from build123d import *

# Parameters (mm, degrees)
SKETCH_W        = 190
SKETCH_H        = 300
PAD_DEPTH       = 6.35
SKETCH001_R     = 2.75
POCKET_DEPTH    = 6.351
SKETCH002_R     = 4
SKETCH002_W     = 10
SKETCH002_H     = 4.75
SKETCH002_W_2   = 4.75
SKETCH002_H_2   = 10
POCKET001_DEPTH = 6.351
SKETCH003_R     = 4
POCKET002_DEPTH = 6.351
SKETCH004_R     = 2.5781
POCKET003_DEPTH = 6.351


with BuildPart() as part:
    # Sketch → Pad (new body)
    with BuildSketch(Plane.XY):
        with Locations((95, 150)):
            Rectangle(SKETCH_W, SKETCH_H)
    extrude(amount=PAD_DEPTH)

    # Sketch001 → Pocket (cut, through all)
    with BuildSketch(Plane.XY.offset(6.35)):
        with Locations((20, 280)):
            Circle(SKETCH001_R)
        with Locations((20, 240)):
            Circle(SKETCH001_R)
        with Locations((60, 240)):
            Circle(SKETCH001_R)
        with Locations((60, 280)):
            Circle(SKETCH001_R)
        with Locations((128, 280)):
            Circle(SKETCH001_R)
        with Locations((168, 280)):
            Circle(SKETCH001_R)
        with Locations((128, 240)):
            Circle(SKETCH001_R)
        with Locations((168, 240)):
            Circle(SKETCH001_R)
        with Locations((20, 55)):
            Circle(SKETCH001_R)
        with Locations((60, 55)):
            Circle(SKETCH001_R)
        with Locations((20, 15)):
            Circle(SKETCH001_R)
        with Locations((60, 15)):
            Circle(SKETCH001_R)
        with Locations((128, 15)):
            Circle(SKETCH001_R)
        with Locations((168, 55)):
            Circle(SKETCH001_R)
        with Locations((128, 55)):
            Circle(SKETCH001_R)
        with Locations((168, 15)):
            Circle(SKETCH001_R)
    extrude(amount=-POCKET_DEPTH, mode=Mode.SUBTRACT)

    # Sketch002 → Pocket001 (cut, through all)
    with BuildSketch(Plane(origin=(0, 0, 0), x_dir=(1, 0, 0), z_dir=(0, 0, -1))):
        with Locations((49.875, -148)):
            Circle(SKETCH002_R)
        with Locations((49.875, -192)):
            Circle(SKETCH002_R)
        with Locations((140.125, -148)):
            Circle(SKETCH002_R)
        with Locations((140.125, -192)):
            Circle(SKETCH002_R)
        with Locations((95, -122.375)):
            Rectangle(SKETCH002_W, SKETCH002_H)
        with Locations((95, -217.375)):
            Rectangle(SKETCH002_W, SKETCH002_H)
        with Locations((49.875, -170)):
            Rectangle(SKETCH002_W_2, SKETCH002_H_2)
        with Locations((140.125, -170)):
            Rectangle(SKETCH002_W_2, SKETCH002_H_2)
    extrude(amount=-POCKET001_DEPTH, mode=Mode.SUBTRACT)

    # Sketch003 → Pocket002 (cut, through all)
    with BuildSketch(Plane(origin=(0, 0, 0), x_dir=(1, 0, 0), z_dir=(0, 0, -1))):
        with Locations((73, -217.375)):
            Circle(SKETCH003_R)
        with Locations((117, -217.375)):
            Circle(SKETCH003_R)
        with Locations((73, -122.375)):
            Circle(SKETCH003_R)
        with Locations((117, -122.375)):
            Circle(SKETCH003_R)
    extrude(amount=-POCKET002_DEPTH, mode=Mode.SUBTRACT)

    # Sketch004 → Pocket003 (cut, through all)
    with BuildSketch(Plane(origin=(0, 0, 0), x_dir=(1, 0, 0), z_dir=(0, 0, -1))):
        with Locations((69, -80)):
            Circle(SKETCH004_R)
        with Locations((89, -80)):
            Circle(SKETCH004_R)
        with Locations((89, -100)):
            Circle(SKETCH004_R)
        with Locations((69, -100)):
            Circle(SKETCH004_R)
    extrude(amount=-POCKET003_DEPTH, mode=Mode.SUBTRACT)


solid = part.part
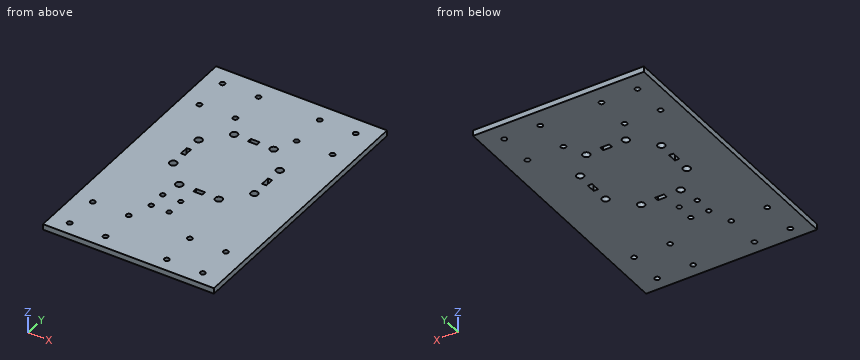
Verification items for the finished model (mm, model axes). Give positions to 0.01 mm unless a question says otherwise; leave off trailing zeros. Write each loop counter-clockwise with the first axis right and the second up, starting at its lowest first coordinate (ties: lowest second). Pieces come first, ordered by that corner, then holes. Notation, with made-up numbers: M 30,-20 L 75,-20 A27 cw 75,14 Z; hole C 50.5,-15.75 d4. An arc over 180 degrees is marked long. Write item = value, one per line.
(1) Go/stop test with flat-tipped pins: pin 1 Ø2 at (y, z) = (139.5, 1) entering from -X; pin 2 Ø3.5 at (x, y) = (128, 280) entering from +Z. Record where each tip stops, or that it passes through.
Found:
pin_1 = 0
pin_2 = through
(2) Sectioned sample at B-B (x = 95). Record the cut outline in (y, z).
Found:
outline = M 0,0 L 120,0 L 120,6.35 L 0,6.35 Z; M 124.75,0 L 215,0 L 215,6.35 L 124.75,6.35 Z; M 219.75,0 L 300,0 L 300,6.35 L 219.75,6.35 Z
(3) Material ranges on line 1 (X direction, y = 80, z = 1.25); line 2 (X direction, y = 280, z = 1.5); line 3 (Y direction, x = 97, z = 6), recorded low to high.
Found:
line_1 = 0 to 66.42, 71.58 to 86.42, 91.58 to 190
line_2 = 0 to 17.25, 22.75 to 57.25, 62.75 to 125.25, 130.75 to 165.25, 170.75 to 190
line_3 = 0 to 120, 124.75 to 215, 219.75 to 300
(4) Sectioned sample at A-A (y = 148). Record the cut outline in (x, z) (3 decimals), then the cut area to 3 significant figures.
Found:
outline = M 0,0 L 45.875,0 L 45.875,6.35 L 0,6.35 Z; M 53.875,0 L 136.125,0 L 136.125,6.35 L 53.875,6.35 Z; M 144.125,0 L 190,0 L 190,6.35 L 144.125,6.35 Z
area = 1,100 mm2
(5) Sectioned sample at C-C (z = 3.25). Give the number of separate pieces and of enclosed holes in the cut face, then the cut area to 3 significant figures.
Found:
separate_pieces = 1
enclosed_holes = 32
area = 55,900 mm2
